Part model, mm, in its own coordinate system. A direction names the side the tool comes from. Give positions to 0.01 mm unless a question says otherwise; leave off trailing zeros. Write each loop counter-clockwise with the first axis right and the second up, starting at its lowest first coordinate (ties: lowest second). Pieces come first, ordered by that corner, then holes. Notation, with made-up numbers: (24, 21) - (58, 21) arc R14 cw to (58, 45) - close; hole circle Ø2 at (29, 79.25). An arc over 180 degrees is marked (long way). Answer in a Markdown table with one row per item. Add a question column.
1. Band-saw the part on A-A on y = -27. Write the cut outline in (x, z) (3 decimals).
2. Band-saw the part on B-B on y = -45.5. Write the cut outline in (x, z) (3 decimals).
3. Probe line 1 along X through (y, z) = (-5.5, -2); line 2 along Z through (x, y) = (44.5, -32.5); line 3 along Z through (x, y) = (-53, -28.5). List the from-to ranges inside material, lowest first.
4. Band-saw the part on D-D on y = -18.5. Write the cut outline in (x, z) (3 decimals).
5. Pull direction Z, two halves, no side cores. Call faces 4 (the flat face through (0, -25.4, 0)), 5 (the flat face through (9.871, -12.522, 21.015)), 6 (the cylindrical face through (54.41, -18.78, 2.86)), 7 (the flat face through (-46, -25, -3.703)): released by +Z, released by -Z, zero draft, split by the parting line, or undercut.
6. Band-saw the part on C-C on z = 8. Write the cut outline in (x, y).
7. Drop flat-ended pins along their axis: pin 1 Ø1.1 at (x, y) = (-46.5, -24) entering from -Z; pin 2 Ø1 at (x, y) = (28.5, -21) entering from +Z; pin 3 Ø2 at (y, z) = (-13, -1.5) entering from -X; pin 4 Ø15 at (x, z) = (45.32, 0) entering from -Y (3 decimals). Give the stop position or say it passes through.
8. Which spindle directions (+Z, -Z, +X, -X, +Y, -Y) get a long thin tool onto all of the face, cutting with end or side? Do faces 1 (the flat face through (-35, 0, 1)), 2 (the flat face through (56, -38.1, 0)), 3 (the flat face through (-68.551, -25, 0)). Say none if no direction does.
```python
from build123d import *

# Parameters (mm, degrees)
F0_R     = 9.525
F1_DEPTH = 25.4
F2_DEPTH = 50.03695
F3_DEPTH = 38.1


with BuildPart() as f1:
    # F0 (on Front) → F1 (new body)
    with BuildSketch(Plane.XZ):
        with BuildLine():
            ThreePointArc((-28.862271, 26.460221), (-20.947828, 14.268476), (-18.175163, 0))
            ThreePointArc((-18.175163, 0), (-20.947828, -14.268476), (-28.862271, -26.460221))
            Line((-28.862271, -26.460221), (47.534793, -15.720424))
            ThreePointArc((47.534793, -15.720424), (29.449837, 0), (47.534793, 15.720424))
            Line((47.534793, 15.720424), (-28.862271, 26.460221))
        make_face()
        with BuildLine():
            ThreePointArc((61.199837, 0), (57.306044, 10.414715), (47.534793, 15.720424))
            ThreePointArc((47.534793, 15.720424), (29.449837, 0), (47.534793, -15.720424))
            ThreePointArc((47.534793, -15.720424), (57.306044, -10.414715), (61.199837, 0))
        make_face()
        with Locations((45.324837, 0)):
            Circle(F0_R, mode=Mode.SUBTRACT)
        with BuildLine():
            ThreePointArc((-28.862271, -26.460221), (-20.947828, -14.268476), (-18.175163, 0))
            ThreePointArc((-18.175163, 0), (-20.947828, 14.268476), (-28.862271, 26.460221))
            ThreePointArc((-28.862271, 26.460221), (-94.375163, 0), (-28.862271, -26.460221))
        make_face()
        with BuildLine():
            ThreePointArc((-65.050929, 3.702913), (-56.275163, 9.525), (-47.499398, 3.702913))
            Line((-47.499398, 3.702913), (-43.999273, 3.702913))
            Line((-43.999273, 3.702913), (-43.999273, -3.702913))
            Line((-43.999273, -3.702913), (-47.499398, -3.702913))
            ThreePointArc((-47.499398, -3.702913), (-56.275163, -9.525), (-65.050929, -3.702913))
            Line((-65.050929, -3.702913), (-68.551053, -3.702913))
            Line((-68.551053, -3.702913), (-68.551053, 3.702913))
            Line((-68.551053, 3.702913), (-65.050929, 3.702913))
        make_face(mode=Mode.SUBTRACT)
    extrude(amount=F1_DEPTH)

    # F0 (on Front) → F2 (join)
    with BuildSketch(Plane.XZ):
        with BuildLine():
            ThreePointArc((-28.862271, -26.460221), (-20.947828, -14.268476), (-18.175163, 0))
            ThreePointArc((-18.175163, 0), (-20.947828, 14.268476), (-28.862271, 26.460221))
            ThreePointArc((-28.862271, 26.460221), (-94.375163, 0), (-28.862271, -26.460221))
        make_face()
        with BuildLine():
            ThreePointArc((-65.050929, 3.702913), (-56.275163, 9.525), (-47.499398, 3.702913))
            Line((-47.499398, 3.702913), (-43.999273, 3.702913))
            Line((-43.999273, 3.702913), (-43.999273, -3.702913))
            Line((-43.999273, -3.702913), (-47.499398, -3.702913))
            ThreePointArc((-47.499398, -3.702913), (-56.275163, -9.525), (-65.050929, -3.702913))
            Line((-65.050929, -3.702913), (-68.551053, -3.702913))
            Line((-68.551053, -3.702913), (-68.551053, 3.702913))
            Line((-68.551053, 3.702913), (-65.050929, 3.702913))
        make_face(mode=Mode.SUBTRACT)
    extrude(amount=F2_DEPTH)

    # F0 (on Front) → F3 (join)
    with BuildSketch(Plane.XZ):
        with BuildLine():
            ThreePointArc((61.199837, 0), (57.306044, 10.414715), (47.534793, 15.720424))
            ThreePointArc((47.534793, 15.720424), (29.449837, 0), (47.534793, -15.720424))
            ThreePointArc((47.534793, -15.720424), (57.306044, -10.414715), (61.199837, 0))
        make_face()
        with Locations((45.324837, 0)):
            Circle(F0_R, mode=Mode.SUBTRACT)
    extrude(amount=F3_DEPTH)


solid = f1.part
```
Values:
| question | item | result |
|---|---|---|
| 1 | outline | (-28.862, -26.46) arc R38.1 ccw to (-18.175, 0) arc R38.1 ccw to (-28.862, 26.46) arc R38.1 ccw (long way) to start; (47.535, -15.72) arc R15.875 ccw to (61.2, 0) arc R15.875 ccw to (47.535, 15.72) arc R15.875 ccw (long way) to start; hole (-68.551, -3.703) - (-65.051, -3.703) arc R9.525 ccw to (-47.499, -3.703) - (-43.999, -3.703) - (-43.999, 3.703) - (-47.499, 3.703) arc R9.525 ccw to (-65.051, 3.703) - (-68.551, 3.703) - close; hole circle Ø19.05 at (45.325, 0) |
| 2 | outline | (-28.862, -26.46) arc R38.1 ccw to (-18.175, 0) arc R38.1 ccw to (-28.862, 26.46) arc R38.1 ccw (long way) to start; hole (-68.551, -3.703) - (-65.051, -3.703) arc R9.525 ccw to (-47.499, -3.703) - (-43.999, -3.703) - (-43.999, 3.703) - (-47.499, 3.703) arc R9.525 ccw to (-65.051, 3.703) - (-68.551, 3.703) - close |
| 3 | line 1 | x = -94.32 to -68.55, -44 to 36.01, 54.64 to 61.07 |
| 3 | line 2 | z = -15.85 to -9.49, 9.49 to 15.85 |
| 3 | line 3 | z = -37.96 to -8.94, 8.94 to 37.96 |
| 4 | outline | (-28.862, -26.46) - (47.535, -15.72) arc R15.875 ccw to (61.2, 0) arc R15.875 ccw to (47.535, 15.72) - (-28.862, 26.46) arc R38.1 ccw (long way) to start; hole (-68.551, -3.703) - (-65.051, -3.703) arc R9.525 ccw to (-47.499, -3.703) - (-43.999, -3.703) - (-43.999, 3.703) - (-47.499, 3.703) arc R9.525 ccw to (-65.051, 3.703) - (-68.551, 3.703) - close; hole circle Ø19.05 at (45.325, 0) |
| 5 | face 4 | zero draft |
| 5 | face 5 | released by +Z |
| 5 | face 6 | undercut |
| 5 | face 7 | undercut |
| 6 | outline | (-93.53, -50.04) - (-61.44, -50.04) - (-61.44, 0) - (-93.53, 0) - close; (-51.11, -50.04) - (-19.02, -50.04) - (-19.02, -25.4) - (31.61, -25.4) - (31.61, -38.1) - (40.16, -38.1) - (40.16, 0) - (-51.11, 0) - close; (50.49, -38.1) - (59.04, -38.1) - (59.04, 0) - (50.49, 0) - close |
| 7 | pin 1 | stops at z = -36.97 |
| 7 | pin 2 | stops at z = 18.47 |
| 7 | pin 3 | stops at x = -94.37 |
| 7 | pin 4 | passes through |
| 8 | face 1 | +Z, -Z, +X, -X, +Y |
| 8 | face 2 | +Z, -Z, +X, -Y |
| 8 | face 3 | +Y, -Y |
